Geometry: final body of the model. Coordinates: model frame, mm. Round coordinates to 2 decimals unless told otherwise and drop trailing zeros. Loops run counter-clockwise (first coordinate to the right, second up) from the corner with the lowest first, then second, coordinate; pieces in that order, holes last. Notation, with made-up numbers: (59.25, -27) -> (93.25, -27) arc R19 ccw to (93.25, -14) -> close; hole circle Ø5 at (46.25, 45.5). An arc over 180 degrees is marked (long way). Answer in a Markdown table with one row per item.
```python
from build123d import *

# Parameters (mm, degrees)
SKETCH018_R      = 11
EXTRUDE016_DEPTH = 11
SKETCH015_W      = 33.86
SKETCH015_H      = 26.75
SKETCH015_R      = 1.65
EXTRUDE017_DEPTH = 1.6
SKETCH016_W      = 17
SKETCH016_H      = 12.75
EXTRUDE018_DEPTH = 4.3
SKETCH017_R      = 13.61
EXTRUDE015_DEPTH = 19.27
SKETCH028_W      = 94
SKETCH028_H      = 54
SKETCH028_R      = 1.65
SKETCH028_W_2    = 40
SKETCH028_H_2    = 40
EXTRUDE028_DEPTH = 2


with BuildPart() as extrude_joystick_stick:
    # Sketch018 → Extrude016 (new body)
    with BuildSketch(Plane.XY):
        with Locations((16.975, 14)):
            Circle(SKETCH018_R)
    extrude(amount=EXTRUDE016_DEPTH)


with BuildPart() as extrude_joystick_stick_1:
    # Extrude016 placement: moved
    add(extrude_joystick_stick.part.moved(Location((0, 0, 20.87))))


with BuildPart() as extrude_joystick_base:
    # Sketch015 → Extrude017 (new body)
    with BuildSketch(Plane.XY):
        with Locations((16.93, 13.375)):
            Rectangle(SKETCH015_W, SKETCH015_H)
        with Locations((5, 22.88)):
            Circle(SKETCH015_R, mode=Mode.SUBTRACT)
        with Locations((31.01, 22.88)):
            Circle(SKETCH015_R, mode=Mode.SUBTRACT)
        with Locations((4.99, 3.31)):
            Circle(SKETCH015_R, mode=Mode.SUBTRACT)
        with Locations((31.01, 3.31)):
            Circle(SKETCH015_R, mode=Mode.SUBTRACT)
    extrude(amount=EXTRUDE017_DEPTH)


with BuildPart() as extrude_joystick_connector:
    # Sketch016 → Extrude018 (new body)
    with BuildSketch(Plane.XY):
        with Locations((-8.5, 13.875)):
            Rectangle(SKETCH016_W, SKETCH016_H)
    extrude(amount=EXTRUDE018_DEPTH)


with BuildPart() as extrude_joystick_connector_1:
    # Extrude018 placement: moved
    add(extrude_joystick_connector.part.moved(Location((0.1, 0, 1.6))))


with BuildPart() as fusion_joystick_connector001:
    # Sketch017 → Extrude015 (new body)
    with BuildSketch(Plane.XY):
        with Locations((17.15, 13.61)):
            Circle(SKETCH017_R)
    extrude(amount=EXTRUDE015_DEPTH)


with BuildPart() as fusion_joystick_connector001_1:
    # Extrude015 placement: moved
    add(fusion_joystick_connector001.part.moved(Location((0, 0, 1.6))))

    # Fusion005: union Extrude_JoyStick_Stick, Extrude_JoyStick_base, Extrude_JoyStick_connector
    add(extrude_joystick_stick_1.part)
    add(extrude_joystick_base.part)
    add(extrude_joystick_connector_1.part)


with BuildPart() as fusion_joystick_connector001_2:
    # Fusion005 placement: moved
    add(fusion_joystick_connector001_1.part.moved(Location((53, 5, 5))))


with BuildPart() as cut_controllercase_top:
    # Sketch028 → Extrude028 (new body)
    with BuildSketch(Plane.XY):
        with Locations((45, 25)):
            Rectangle(SKETCH028_W, SKETCH028_H)
        with Locations((1, 49)):
            Circle(SKETCH028_R, mode=Mode.SUBTRACT)
        with Locations((89, 49)):
            Circle(SKETCH028_R, mode=Mode.SUBTRACT)
        with Locations((89, 1)):
            Circle(SKETCH028_R, mode=Mode.SUBTRACT)
        with Locations((1, 1)):
            Circle(SKETCH028_R, mode=Mode.SUBTRACT)
        with Locations((25, 25)):
            Rectangle(SKETCH028_W_2, SKETCH028_H_2, mode=Mode.SUBTRACT)
    extrude(amount=EXTRUDE028_DEPTH)


with BuildPart() as cut_controllercase_top_1:
    # Extrude028 placement: moved
    add(cut_controllercase_top.part.moved(Location((0, 0, 19))))

    # Cut003: cut Fusion_JoyStick_connector001
    add(fusion_joystick_connector001_2.part, mode=Mode.SUBTRACT)


solid = cut_controllercase_top_1.part
```
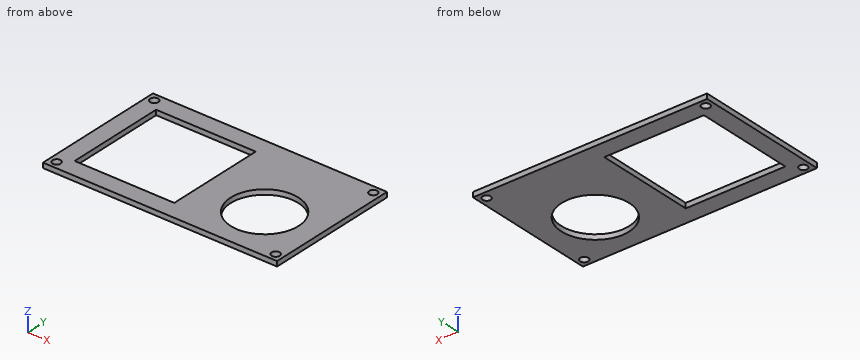
Item 1: Ray query, L1, parallel to Y at x = 89, z = 20.55; L2, parallel to X at y = 7.5, z = 19.9; L3, parallel to Y at x = 26, z = 20.45. Return the intervals inside material, ascending.
Ans:
| item | result |
|---|---|
| L1 | -2 to -0.65, 2.65 to 47.35, 50.65 to 52 |
| L2 | -2 to 5, 45 to 62.29, 78.01 to 92 |
| L3 | -2 to 5, 45 to 52 |
Item 2: Section query D-D, the plane y = 1. Output: boundary loops of the cut face in (x, z).
Ans:
| item | result |
|---|---|
| outline | (-2, 19) -> (-0.65, 19) -> (-0.65, 21) -> (-2, 21) -> close; (2.65, 19) -> (87.35, 19) -> (87.35, 21) -> (2.65, 21) -> close; (90.65, 19) -> (92, 19) -> (92, 21) -> (90.65, 21) -> close |
Item 3: Section query C-C, the plane x = 89. Output: boundary loops of the cut face in (y, z), and give its area (3 significant figures).
Ans:
| item | result |
|---|---|
| outline | (-2, 19) -> (-0.65, 19) -> (-0.65, 21) -> (-2, 21) -> close; (2.65, 19) -> (47.35, 19) -> (47.35, 21) -> (2.65, 21) -> close; (50.65, 19) -> (52, 19) -> (52, 21) -> (50.65, 21) -> close |
| area | 94.8 mm2 |
Item 4: First-contact query: P1, Ø10, axis at x = 14.5, y = 11.5, coming from the +Z side (3 decimals). Flat tip, straight axial feed; report the tip coordinate or a pass-through.
Ans:
| item | result |
|---|---|
| P1 | through |
Item 5: Section query A-A, the plane y = 35. Output: boundary loops of the cut face in (x, z).
Ans:
| item | result |
|---|---|
| outline | (-2, 19) -> (5, 19) -> (5, 21) -> (-2, 21) -> close; (45, 19) -> (92, 19) -> (92, 21) -> (45, 21) -> close |
Item 6: Section query B-B, the plane x = 19.5. Output: boundary loops of the cut face in (y, z).
Ans:
| item | result |
|---|---|
| outline | (-2, 19) -> (5, 19) -> (5, 21) -> (-2, 21) -> close; (45, 19) -> (52, 19) -> (52, 21) -> (45, 21) -> close |
